Autodesk Inventor part; units mm, degrees
ref_plane "YZ Plane" through (0, 0, 0) normal (1, 0, 0) x (0, 1, 0)
ref_plane "XZ Plane" through (0, 0, 0) normal (0, 1, 0) x (-1, 0, 0)
ref_plane "XY Plane" through (0, 0, 0) normal (0, 0, 1) x (1, 0, 0)
sketch "Sketch1" plane through (0, 0, 0) normal (1, 0, 0) x (0, 1, 0)
  line L0 (0, 0) -> (750, 0)
  line L1 (750, 0) -> (750, -750)
  line L2 (750, -750) -> (0, -750)
  line L3 (0, -750) -> (0, 0)
  dimension "d0" = 750
  dimension "d1" = 750
extrude "Extrusion1" add sketch "Sketch1" along normal blind 1000
sketch "Sketch2" plane through (1000, 0, 0) normal (1, 0, 0) x (0, 0, -1)
  line L0 (750, 0) -> (750, 750)
  line L1 (0, 0) -> (750, 0)
  circle A0 centre (374.0764, 375) radius 250
  dimension "d4" = 500
extrude "Extrusion2" cut sketch "Sketch2" against normal blind 750
sketch "Sketch3" plane through (250, 375, -374.0764) normal (1, 0, 0) x (0, 0, -1)
  line L0 (0, 0) -> (-100, 0)
  line L1 (0, 0) -> (100, 0)
  circle A0 centre (100, 0) radius 50
  circle A1 centre (-100, 0) radius 50
  point P0 (-374.0764, -375)
  dimension "d7" = 100
  dimension "d8" = 100
  dimension "d9" = 100
  dimension "d10" = 100
extrude "Extrusion3" add sketch "Sketch3" along normal blind 50
chamfer "Chamfer1" distance 50 angle 45 1 edges at (250, 375, -124.0764)
chamfer "Chamfer2" distance 50 angle 45 1 edges at (1000, 375, -124.0764)
sketch "Sketch4" plane through (300, 375, -274.0764) normal (1, 0, 0) x (0, 0, -1)
  line L0 (0, 0) -> (0, -19)
  line L1 (0, -19) -> (-30, -19)
  line L2 (0, -19) -> (30, -19)
  line L3 (30, -19) -> (30, 0)
  line L4 (30, 0) -> (-30, 0)
  line L5 (-30, 0) -> (-30, -19)
  line L6 (195.1877, 10) -> (195.1877, 30)
  line L7 (195.1877, 30) -> (205.1877, 30)
  line L8 (205.1877, -30) -> (195.1877, -30)
  line L9 (195.1877, -30) -> (195.1877, -10)
  line L10 (205.1877, 30) -> (205.1877, 10)
  line L11 (205.1877, -30) -> (205.1877, -10)
  line L12 (195.1877, -10) -> (195.1877, -5)
  line L13 (195.1877, -5) -> (170.1877, -5)
  line L14 (170.1877, -5) -> (170.1877, 5)
  line L15 (170.1877, 5) -> (195.1877, 5)
  line L16 (195.1877, 10) -> (195.1877, 5)
  line L17 (205.1877, 10) -> (205.1877, 5)
  line L18 (205.1877, 5) -> (230.1877, 5)
  line L19 (205.1877, -10) -> (205.1877, -5)
  line L20 (205.1877, -5) -> (230.1877, -5)
  line L21 (230.1877, 5) -> (230.1877, -5)
  point P0 (-274.0764, -375)
  dimension "d19" = 19
  dimension "d20" = 30
  dimension "d21" = 30
  dimension "d27" = 20
  dimension "d28" = 10
  dimension "d29" = 60
  dimension "d30" = 5
  dimension "d31" = 10
extrude "Extrusion4" cut sketch "Sketch4" against normal blind 10
properties part number "heavy lithium cell receptical"
Work out the finished part from the listing and answer in its coordinate system (mm). A direction names the side the tool comes from. Give positions to 0.01 mm unless a question says otherwise; leave off trailing zeros. Loops run counter-clockwise (first coordinate to the right, second up) from the corner with the lowest first, then second, coordinate; pieces in that order, holes last. Notation, with made-up numbers: (-36, 75.25) -> (-7, 75.25) arc R24 ccw to (-7, 94.25) -> close; hole circle Ø11 at (47, 77). An arc over 180 degrees is marked (long way). Use a Markdown table: item, result. Add a question column.
1. Determine the mould class of faces 3 (the flat face through (493, 0, -380)), 4 (the cylindrical face through (274.65, 325.425, -467.567)), 5 (the flat face through (493, 370, 0)) for opening direction Z: released by +Z, released by -Z, zero draft, split by the parting line, or undercut.
2. Section A-A on x = 497 is taken. Determine the outline of the cut face in (y, z), and give its area (3 significant figures).
3. For faces 1 (the flat face through (493, 750, -370)), 2 (the cylindrical face through (629.55, 279.249, -605.013)), determine the directions among +Z, -Z, +X, -X, +Y, -Y from which every point of the face is accessible in a straight line to the end or side of a thin tool.
4. Flat-ended cylindrical pins translate along their axes: pin 1 Ø9.5 at (y, z) = (362.5, -278) entering from +X; pin 2 Ø18 at (y, z) = (368, -482.5) entering from +X. Find the tip coordinate at first contact, or state that the pin passes through.
5. Find the intervals of material crossed by probe 1 along X at (y, z) = (293.5, -451.5); probe 2 along Z at (x, y) = (617.5, 261.5); probe 3 along Y at (x, z) = (912.5, -445), in increasing order.
Results below:
| question | item | result |
|---|---|---|
| 1 | face 3 | zero draft |
| 1 | face 4 | undercut |
| 1 | face 5 | released by +Z |
| 2 | outline | (0, -750) -> (750, -750) -> (750, 0) -> (0, 0) -> close; hole circle Ø500 at (375, -374.08) |
| 2 | area | 366,000 mm^2 |
| 3 | face 1 | +Z, -Z, +X, -X, +Y |
| 3 | face 2 | +X |
| 4 | pin 1 | stops at x = 290 |
| 4 | pin 2 | stops at x = 300 |
| 5 | probe 1 | x = 0 to 250 |
| 5 | probe 2 | z = -750 to -596.83, -151.33 to 0 |
| 5 | probe 3 | y = 0 to 135.27, 614.73 to 750 |
